The model under review builds one solid part; all positions refer to its coordinate system, in mm. A direction names the side the tool comes from. Coordinates: 2 decimals unless noted, no trailing zeros. Order: outer loops, then holes, each group sorted by start corner. A loop starts at its lowest first (then second) coordinate and runs counter-clockwise, first axis right, second up. Notation, with made-up numbers: (-32, -24) -> (1, -24) arc R21 cw to (1, -2) -> close; hole circle Ø3 at (88.25, -9.75). An arc over 180 degrees is marked (long way). Use one line per item in the form item = value. Start each with the question number.
(1) Take a section at A-A (y = 0). State the section outline as (x, z) points, then the cut area to 3 significant figures.
(2) Insertion check: pin 1 Ø1.5 at (y, z) = (-2, 1) entering from +X; pin 2 Ø3.5 at (x, y) = (0, 0) entering from +Z; pin 3 Ø0.5 at (x, z) = (-4, 4) entering from -Y. Each pin has a flat end and moves straight along its axis. Give the tip position at first contact, or say it passes through.
(3) For faces 1 (the flat face through (1, -4, 4.6)), 2 (the flat face through (0.942, 4.606, 4.107)), list the 3-axis set-ups (+Z, -Z, +X, -X, +Y, -Y) from which the entire face can be reached by the end or side of a thin tool; tool diameter is ignored.
(4) Wall thickness on line 1 along Y through (x, z) = (0, 2.4); line 2 along Z through (x, y) = (7.25, 6.25); line 3 along Z through (x, y) = (-1.75, -2.5): over which ranges is each line inside the solid? List them lowest first.
(5) Take a section at B-B (z = 2.95). State the section outline as (x, y) points, then the cut area to 3 significant figures.
(6) Mouldability with a two-part tool opening along X and no side actions: class faces 3 (the flat face through (4.533, 0.011, 4.107)), 4 (the flat face through (2, 0, 0)), 5 (the cylindrical face through (6.466, 2.681, 2.424)) as +X half, -X half, draft (parallel to the pull), parting line (faces both ways), or undercut.
Solid Edge part; units mm, degrees
sketch "Sketch1" plane through (0, 0, 0) normal (0, 0, 1) x (1, 0, 0)
  circle A0 centre (0, 0) radius 10
extrude "Protrusion1" add sketch "Sketch1" along normal blind 0.6
sketch "Sketch2" plane through (0, 0, 0.6) normal (0, 0, 1) x (1, 0, 0)
  circle A0 centre (0, 0) radius 7
extrude "ExtrudedProtrusion_2" add sketch "Sketch2" along normal blind 4
fillet "Round_1" radius 0.3 1 edges at (-7, 0, 4.6)
fillet "Round_2" radius 0.2 1 edges at (-10, 0, 0.6)
sketch "Sketch3" plane through (0, 0, 4.6) normal (0, 0, 1) x (1, 0, 0)
  line L0 (3.5912, 0.8017) -> (5.5021, -0.8017)
  line L1 (5.5021, -0.8017) -> (3.1581, -1.6548)
  line L2 (3.1581, -1.6548) -> (3.5912, -4.1114)
  line L3 (3.5912, -4.1114) -> (1.2472, -3.2582)
  line L4 (0, -5.4185) -> (1.2472, -3.2582)
  line L5 (-1.2472, -3.2582) -> (0, -5.4185)
  line L6 (-1.2472, -3.2582) -> (-3.5912, -4.1114)
  line L7 (-3.5912, -4.1114) -> (-3.1581, -1.6548)
  line L8 (-3.1581, -1.6548) -> (-5.5021, -0.8017)
  line L9 (-5.5021, -0.8017) -> (-3.5912, 0.8017)
  line L10 (-4.8384, 2.9619) -> (-3.5912, 0.8017)
  line L11 (-2.344, 2.9619) -> (-4.8384, 2.9619)
  line L12 (-2.344, 2.9619) -> (-1.9108, 5.4185)
  line L13 (-1.9108, 5.4185) -> (0, 3.8151)
  line L14 (0, 3.8151) -> (1.9108, 5.4185)
  line L15 (1.9108, 5.4185) -> (2.344, 2.9619)
  line L16 (4.8384, 2.9619) -> (2.344, 2.9619)
  line L17 (3.5912, 0.8017) -> (4.8384, 2.9619)
extrude "ExtrudedCutout_1" cut sketch "Sketch3" against normal blind 1
sketch "Sketch4" plane through (0, 0, 0) normal (0, 0, -1) x (1, 0, 0)
  circle A0 centre (0, 0) radius 1.35
extrude "ExtrudedCutout_2" cut sketch "Sketch4" against normal blind 5
Findings:
q1.outline = (-10, 0) -> (-1.35, 0) -> (-1.35, 3.6) -> (-4.55, 3.6) -> (-4.55, 4.6) -> (-6.7, 4.6) arc R0.3 ccw to (-7, 4.3) -> (-7, 0.6) -> (-9.8, 0.6) arc R0.2 ccw to (-10, 0.4) -> close; (1.35, 0) -> (10, 0) -> (10, 0.4) arc R0.2 ccw to (9.8, 0.6) -> (7, 0.6) -> (7, 4.3) arc R0.3 ccw to (6.7, 4.6) -> (4.55, 4.6) -> (4.55, 3.6) -> (1.35, 3.6) -> close
q1.area = 49.1 mm²
q2.pin_1 = 9.88
q2.pin_2 = 3.6
q2.pin_3 = -5.91
q3.face_1 = +Z, +X, -X, +Y, -Y
q3.face_2 = +Z
q4.line_1 = -7 to -1.35, 1.35 to 7
q4.line_2 = 0 to 0.6
q4.line_3 = 0 to 3.6
q5.outline = circle Ø14 at (0, 0); hole circle Ø2.7 at (0, 0)
q5.area = 148 mm²
q6.face_3 = undercut
q6.face_4 = draft
q6.face_5 = parting line
